Autodesk Inventor part; units mm, degrees
ref_plane "YZ Plane" through (0, 0, 0) normal (1, 0, 0) x (0, 1, 0)
ref_plane "XZ Plane" through (0, 0, 0) normal (0, 1, 0) x (-1, 0, 0)
ref_plane "XY Plane" through (0, 0, 0) normal (0, 0, 1) x (1, 0, 0)
sketch "Sketch1" plane through (0, 0, 0) normal (0, 1, 0) x (-1, 0, 0)
  line L0 (0, -53.34) -> (0, 53.34)
  line L1 (-24.5, 0) -> (24.5, 0)
  line L2 (24.5, 0) -> (-24.5, 0)
  line L3 (0, -53.34) -> (0, 53.34)
  line L4 (-17.5, 38.1) -> (-17.5, -38.1)
  line L5 (-17.5, -38.1) -> (17.5, -38.1)
  line L6 (17.5, -38.1) -> (17.5, 38.1)
  line L7 (17.5, 38.1) -> (-17.5, 38.1)
  line L8 (-17.5, -38.1) -> (17.5, 38.1) construction
  point P0 (0, 0)
  dimension "d1" = 76.2
  dimension "d2" = 35
extrude "Extrusion1" add sketch "Sketch1" along normal mid plane 20
sketch "Sketch2" plane through (0, 10, 0) normal (0, 1, 0) x (1, 0, 0)
  point P0 (0, 0)
  point P1 (0, 0)
hole "Hole1" at (0, 10, 0) direction (0, -1, 0) diameter 28.575 end through all counterbore diameter 31.13 counterbore depth 1.6
fillet "Fillet1" radius 3.175 4 edges at (17.5, 0, 38.1) (17.5, 0, -38.1) (-17.5, 0, 38.1) (-17.5, 0, -38.1)
sketch "Sketch3" plane through (-17.5, -10, -34.925) normal (-1, 0, 0) x (0, 0, 1)
  line L0 (0, 0) -> (0, 20)
  line L1 (69.85, 0) -> (0, 0)
  line L2 (69.85, 20) -> (69.85, 0)
  line L3 (0, 20) -> (69.85, 20)
  line L4 (0, 20) -> (0, 0)
  line L5 (0, 0) -> (69.85, 0)
  line L6 (69.85, 0) -> (69.85, 20)
  line L7 (69.85, 20) -> (0, 20)
  line L8 (0, 20) -> (0, 0)
  line L9 (19.36, 20) -> (50.49, 20)
  line L10 (34.925, 20) -> (34.925, 0)
  line L11 (0, 10) -> (69.85, 10)
  line L12 (69.85, 0) -> (69.85, 20)
  point P0 (34.925, 10)
  point P1 (9.525, 10)
  point P2 (60.325, 10)
  dimension "d19" = 25.4
  dimension "d20" = 25.4
hole "Hole2" at (-17.5, 0, -25.4) at (-17.5, 0, 25.4) direction (1, 0, 0) diameter 4.826 end through all counterbore diameter 7.874 counterbore depth 10.16
properties part number "BearingBlock30mmRight"
Geometry: final body of the model. Coordinates: model frame, mm. A direction names the side the tool comes from. Give positions to 0.01 mm unless a question says otherwise; leave off trailing zeros. Write each loop counter-clockwise with the first axis right and the second up, starting at its lowest first coordinate (ties: lowest second). Pieces come first, ordered by that corner, then holes.
(1) First-contact query: P1, Ø7.5, axis at y = 0, z = 25.4, coming from the -X side; P2, Ø18.5, axis at x = 0, z = 0, coming from the -Y side. Flat tips, straight axial feed; report the tip coordinate or a pass-through.
(2) Mould query, pull axis X, two halves, no side actions, for faces 1 (the flat face through (-7.34, 3, 25)), 2 (the cylindrical face through (15.195, 9.189, -3.374)), 3 (the cylindrical face through (-12.349, -0.173, 21.467)), 4 (the cylindrical face through (-0.628, -0.929, -14.274)). Classes: released by +X, released by -X, zero draft, split by the parting line, or undercut.
(3) Access query for faces 5 (the flat face through (13, 8.4, 7)), 6 (the cylindrical face through (-12.349, 1.508, -21.763)), 7 (the flat face through (0, 0, 38.1)). Directions: +Z, -Z, +X, -X, +Y, -Y. A direction counts if a zero-diameter tool reaches every point of the face in a straight line with its end or side. Return the directions, or none.
(4) Cut plane C-C, the plane z = 0. Return loops of the section in (x, y) (1 decimal).
(5) Cut plane A-A, the plane x = 0. Return loops of the section in (y, z) (1 decimal), then the cut area to 3 significant figures.
(6) Ray query, line 1 (X direction, y = -2, z = 0); line 2 (Y direction, x = 2.5, z = -25.4); line 3 (Z direction, x = 9, y = -2). Return the intervals inside material, ascending.
(7) Cut plane B-B, the plane y = 0. Give the number of separate pieces and of enclosed holes in the cut face, then the cut area to 3 significant figures.
Values follow:
1. P1: stops at x = -7.34
1. P2: passes through
2. face 1: released by -X
2. face 2: undercut
2. face 3: zero draft
2. face 4: undercut
3. face 5: +Y
3. face 6: -X
3. face 7: +Z, +X, -X, +Y, -Y
4. outline: (-17.5, -10) - (-14.3, -10) - (-14.3, 8.4) - (-15.6, 8.4) - (-15.6, 10) - (-17.5, 10) - close; (14.3, -10) - (17.5, -10) - (17.5, 10) - (15.6, 10) - (15.6, 8.4) - (14.3, 8.4) - close
5. outline: (-10, -38.1) - (10, -38.1) - (10, -15.6) - (8.4, -15.6) - (8.4, -14.3) - (-10, -14.3) - close; (-10, 14.3) - (8.4, 14.3) - (8.4, 15.6) - (10, 15.6) - (10, 38.1) - (-10, 38.1) - close; hole circle Ø4.8 at (0, -25.4); hole circle Ø4.8 at (0, 25.4)
5. area: 912 mm2
6. line 1: x = -17.5 to -14.29, 14.29 to 17.5
6. line 2: y = -10 to -2.41, 2.41 to 10
6. line 3: z = -38.1 to -26.75, -24.05 to -11.1, 11.1 to 24.05, 26.75 to 38.1
7. separate pieces: 3
7. enclosed holes: 1
7. area: 1,620 mm2
